Geometry check sheet. Reference: the model listing, model coordinates, mm. A direction names the side the tool comes from. Round coordinates to 2 decimals unless told otherwise and drop trailing zeros. Write each loop counter-clockwise with the first axis right and the second up, starting at its lowest first coordinate (ties: lowest second). Pieces come first, ordered by that corner, then holes. Notation, with made-up numbers: M 53.25,23.25 L 62.25,23.25 A27 cw 62.25,42.25 Z; hole C -27.75,5 d9. An arc over 180 degrees is marked long. Use a Markdown table: item, result.
```python
from build123d import *

# Parameters (mm, degrees)
BOSS_EXTRUDE1_DEPTH = 3
FILLET1_R           = 0.5
SKETCH2_R           = 2.5
CUT_EXTRUDE1_DEPTH  = 4
CUT_EXTRUDE2_DEPTH  = 4
SKETCH4_R           = 1.25
CUT_EXTRUDE3_DEPTH  = 4
CHAMFER1_SIZE       = 0.5


with BuildPart() as part:
    # Sketch1 → Boss-Extrude1 (new body)
    with BuildSketch(Plane(origin=(0, 0, 0), x_dir=(1, 0, 0), z_dir=(0, 1, 0))):
        Polygon((-19.25, 27), (-19.25, -27), (-5, -27), (-5, -28.5), (5, -28.5), (5, -27), (19.25, -27), (19.25, 27), (5, 27), (5, 28.5), (-5, 28.5), (-5, 27), align=None)
    extrude(amount=BOSS_EXTRUDE1_DEPTH)

    # Fillet1
    fillet1_edges = [part.edges().sort_by_distance(p)[0] for p in [
        (0, 0, 28.5),
        (0, 0, -28.5),
    ]]
    fillet(fillet1_edges, radius=FILLET1_R)

    # Sketch2 → Cut-Extrude1 (cut, through all)
    with BuildSketch(Plane(origin=(0, 3, 0), x_dir=(1, 0, 0), z_dir=(0, 1, 0))):
        with Locations((0, -23)):
            Circle(SKETCH2_R)
    extrude(amount=-CUT_EXTRUDE1_DEPTH, mode=Mode.SUBTRACT)

    # Sketch3 → Cut-Extrude2 (cut, through all)
    with BuildSketch(Plane(origin=(0, 3, 0), x_dir=(1, 0, 0), z_dir=(0, 1, 0))):
        with BuildLine():
            Line((-2.1, 28.5), (2.1, 28.5))
            Line((2.1, 28.5), (2.1, 23.2))
            ThreePointArc((2.1, 23.2), (0, 21.1), (-2.1, 23.2))
            Line((-2.1, 23.2), (-2.1, 28.5))
        make_face()
    extrude(amount=-CUT_EXTRUDE2_DEPTH, mode=Mode.SUBTRACT)

    # Sketch4 → Cut-Extrude3 (cut, through all)
    with BuildSketch(Plane(origin=(0, 3, 0), x_dir=(1, 0, 0), z_dir=(0, 1, 0))):
        with Locations((7, -7.25)):
            Circle(SKETCH4_R)
    extrude(amount=-CUT_EXTRUDE3_DEPTH, mode=Mode.SUBTRACT)

    # Chamfer1
    chamfer1_edges = [part.edges().sort_by_distance(p)[0] for p in [
        (5.75, 0, 7.25),
    ]]
    chamfer(chamfer1_edges, length=CHAMFER1_SIZE)


solid = part.part
```
Item 1: Cross-section at C-C, the plane x = 0. Record the cut outline in (y, z).
Outcome:
| item | result |
|---|---|
| outline | M 0,-21.1 L 3,-21.1 L 3,20.5 L 0,20.5 Z; M 0,25.5 L 3,25.5 L 3,28.5 L 0.5,28.5 A0.5 ccw 0,28 Z |
Item 2: Go/stop test with flat-tipped pins: pin 1 (1 mm diameter, centred on x = 13.5, y = 2.5, fed in from -Z); pin 2 (4.5 mm diameter, centred on x = 0, z = 23, fed in from +Y); pin 3 (1.2 mm diameter, centred on y = 1, z = 28, fed in from -X); pin 4 (1.5 mm diameter, centred on x = -15, y = 2, fed in from +Z). Record where each tip stops, or that it passes through.
Outcome:
| item | result |
|---|---|
| pin 1 | stops at z = -27 |
| pin 2 | passes through |
| pin 3 | stops at x = -5 |
| pin 4 | stops at z = 27 |
Item 3: Cross-section at D-D, the plane z = 23. Record the cut outline in (x, y).
Outcome:
| item | result |
|---|---|
| outline | M -19.25,0 L -2.5,0 L -2.5,3 L -19.25,3 Z; M 2.5,0 L 19.25,0 L 19.25,3 L 2.5,3 Z |
Item 4: Access from +Z, -Z, +X, -X, +Y, -Y to the whole of each face (thin tool, end or side, straight path). Record for faces 1 (the face through (5, 1, 28)), 2 (the face through (-5, 1, 28)), 3 (the face through (5, 1, -28)).
Outcome:
| item | result |
|---|---|
| face 1 | +Z, +X, +Y, -Y |
| face 2 | +Z, -X, +Y, -Y |
| face 3 | -Z, +X, +Y, -Y |
Item 5: Mould release check, pull along X, two halves, no side actions. Record for faces 4 (the face through (-19.25, 1, 0)), 5 (the face through (-2.1, 2, -26)), 6 (the face through (0, 0, 0)): +X half, -X half, draft (parallel to the pull), parting line (faces both ways), or undercut.
Outcome:
| item | result |
|---|---|
| face 4 | -X half |
| face 5 | undercut |
| face 6 | draft |
Item 6: Cross-section at A-A, the plane z = 7.25. Record the cut outline in (x, y), and give its area (3 significant figures).
Outcome:
| item | result |
|---|---|
| outline | M -19.25,0 L 5.25,0 L 5.75,0.5 L 5.75,3 L -19.25,3 Z; M 8.25,0.5 L 8.75,0 L 19.25,0 L 19.25,3 L 8.25,3 Z |
| area | 108 mm2 |
Item 7: Cross-section at B-B, the plane y = 1.8. Record the cut outline in (x, z), and give its area (3 significant figures).
Outcome:
| item | result |
|---|---|
| outline | M -19.25,-27 L -5,-27 L -5,-28.5 L -2.1,-28.5 L -2.1,-23.2 A2.1 cw 2.1,-23.2 L 2.1,-28.5 L 5,-28.5 L 5,-27 L 19.25,-27 L 19.25,27 L 5,27 L 5,28.5 L -5,28.5 L -5,27 L -19.25,27 Z; hole C 0,23 d5; hole C 7,7.25 d2.5 |
| area | 2,060 mm2 |
Item 8: Material ranges on line 1 along X through (y, z) = (1.6, 23); line 2 along X through (y, z) = (1.35, 7.25); line 3 along Z through (x, y) = (7, 1.25), recorded low to high. Write a range as from..to.
Outcome:
| item | result |
|---|---|
| line 1 | x = -19.25..-2.5, 2.5..19.25 |
| line 2 | x = -19.25..5.75, 8.25..19.25 |
| line 3 | z = -27..6, 8.5..27 |
